Drawing for the job (mm, zero at the part's lowest x, y, z). A direction names the side the tool comes from. Coordinates: 2 decimals unless noted, no trailing zeros. Write each loop counter-clockwise with the first axis right and the second up, starting at its lowest first coordinate (ties: lowest second). Pieces come first, ordered by that corner, then holes. Notation, with made-up numbers: M -12,-22.75 L 12,-22.75 A12 cw 12,-9.75 Z; hole C 10.5,-24 d11. An arc over 180 degrees is marked long. Use a Markdown table: item, result. Add a question column.
Q1. Wall check: L1, parallel to X at y = 4.25, z = 7.25; L2, parallel to Z at x = 29, y = 4.95. Give the ranges that are in metal, low to high. Write a range as from..to.
Q2. Tool access for the marked faces 1 and 2: list every direction of +Z, -Z, +X, -X, +Y, -Y with a clear straight run to the whole face (end or side of a thin tool).
Q3. Slice it at B-B on y = 1.7. Write the cut outline in (x, z), then the cut area to 3 significant figures.
Q4. Slice it at C-C on x = 33. Write the cut outline in (y, z).
Q5. Pin check, flat tips, straight feed: pin 1 Ø1 at (x, y) = (28.5, 4) entering from -Z; pin 2 Ø4 at (x, z) = (6, 4.5) entering from +Y. Stop position of each tip, or through.
Q6. Slice it at A-A on z = 3.75. Write the cut outline in (x, y), then the cut area to 3 significant figures.
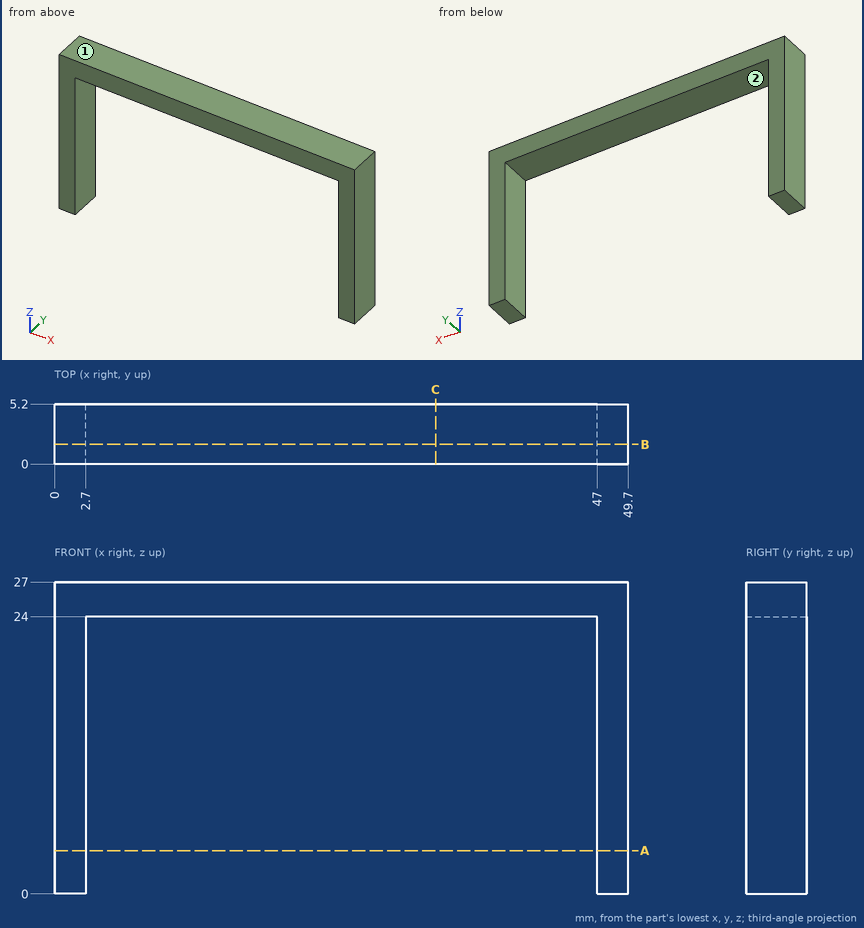
Recorded:
| question | item | result |
|---|---|---|
| 1 | L1 | 0..2.7, 47..49.7 |
| 1 | L2 | 24..27 |
| 2 | face 1 | +Z, +X, -X, +Y, -Y |
| 2 | face 2 | -Z, +Y, -Y |
| 3 | outline | M 0,0 L 2.7,0 L 2.7,24 L 47,24 L 47,0 L 49.7,0 L 49.7,27 L 0,27 Z |
| 3 | area | 279 mm² |
| 4 | outline | M 0,24 L 5.2,24 L 5.2,27 L 0,27 Z |
| 5 | pin 1 | z = 24 |
| 5 | pin 2 | through |
| 6 | outline | M 0,0 L 2.7,0 L 2.7,5.2 L 0,5.2 Z; M 47,0 L 49.7,0 L 49.7,5.2 L 47,5.2 Z |
| 6 | area | 28.1 mm² |
